from build123d import *

# Parameters (mm, degrees)
PAD_DEPTH       = 5.5
SKETCH001_R     = 1.6
POCKET_DEPTH    = 10
CHAMFER_SIZE    = 0.8
FILLET_R        = 2.49
SKETCH002_R     = 20.5
POCKET001_DEPTH = 2.5


with BuildPart() as part:
    # Sketch → Pad (new body)
    with BuildSketch(Plane.XZ):
        Polygon((0, 0), (0, -5), (5.25, -5), (5.25, -1.5), (17.75, -1.5), (17.75, -5), (23, -5), (23, 0), align=None)
    extrude(amount=PAD_DEPTH)

    # Sketch001 → Pocket (cut)
    with BuildSketch(Plane.XY):
        with Locations((2.75, -2.75)):
            Circle(SKETCH001_R)
        with Locations((20.25, -2.75)):
            Circle(SKETCH001_R)
    extrude(amount=-POCKET_DEPTH, mode=Mode.SUBTRACT)

    # Chamfer
    chamfer_edges = [part.edges().sort_by_distance(p)[0] for p in [
        (1.15, -2.75, 0),
        (18.65, -2.75, 0),
    ]]
    chamfer(chamfer_edges, length=CHAMFER_SIZE)

    # Fillet
    fillet_edges = [part.edges().sort_by_distance(p)[0] for p in [
        (0, -5.5, -2.5),
        (0, 0, -2.5),
        (23, 0, -2.5),
        (23, -5.5, -2.5),
        (5.25, -5.5, -3.25),
        (5.25, 0, -3.25),
        (17.75, -5.5, -3.25),
        (17.75, 0, -3.25),
    ]]
    fillet(fillet_edges, radius=FILLET_R)

    # Sketch002 → Pocket001 (cut)
    with BuildSketch(Plane.XY):
        with Locations((11.259596, 20)):
            Circle(SKETCH002_R)
    extrude(amount=-POCKET001_DEPTH, mode=Mode.SUBTRACT)


solid = part.part
CAD build for the part. Positions are in the model's coordinates, mm. A direction names the side the tool comes from. Round coordinates to 2 decimals unless told otherwise and drop trailing zeros. Write each loop counter-clockwise with the first axis right and the second up, starting at its lowest first coordinate (ties: lowest second). Pieces come first, ordered by that corner, then holes. Notation, with made-up numbers: M 76.25,-34 L 90.25,-34 A17 ccw 90.25,-20 Z; hole C -1,24 d2. An arc over 180 degrees is marked long. Use a Markdown table: item, result. Add a question column.
1. Slice it at C-C on z = -0.5. Give the cut face in (x, y), then the cut area to 3 significant figures.
2. 3-axis set-ups, long thin cutter, end or side, ignore diameter. For faces 4 (the face through (4.5, -0.71, -3.23)), 5 (the face through (1, -1, -5)), 6 (the face through (18.5, -4.79, -3.27)): which of +Z, -Z, +X, -X, +Y, -Y reach the whole face in a straight line?
3. Slice it at B-B on z = -4.55. Give the cut face in (x, y).
4. Flat gauge pins, fed straight in: P1, Ø3, axis at x = 2.75, y = -2.75, coming from the +Z side; P2, Ø3, axis at x = 13.5, y = -2, coming from the -Z side. Where does each tip first touch, or does it go through?
5. Drill centre lines: probe 1 along Y at (x, z) = (2.75, -2.1); probe 2 along X at (y, z) = (-4.1, -2.25); probe 3 along Z at (x, y) = (17, -1.5). Where is each one in solid material? Low to high.
6. Pull direction Y, two halves, no side cores. Call faces 1 (the face through (22.29, -0.75, -2.46)), 2 (the face through (22, -4, -5)), 3 (the face through (19.07, -1.67, -2.87)): released by +Y, released by -Y, zero draft, split by the parting line, or undercut.
7. Slice it at A-A on y = -2.75. Give the cut face in (x, z).
8. Slice it at D-D on x = 15. Give the cut face in (y, z), then the cut area to 3 significant figures.
Reply:
| question | item | result |
|---|---|---|
| 1 | outline | M 0,-3.01 A2.49 ccw 2.49,-5.5 L 20.51,-5.5 A2.49 ccw 23,-3.01 L 23,-2.49 A2.49 ccw 20.51,0 L 15.76,0 A20.5 cw 6.76,0 L 2.49,0 A2.49 ccw 0,-2.49 Z; hole C 2.75,-2.75 d3.8; hole C 20.25,-2.75 d3.8 |
| 1 | area | 95.5 mm^2 |
| 2 | face 4 | -Z, +Y |
| 2 | face 5 | -Z, +X, -X, +Y, -Y |
| 2 | face 6 | -Z, -Y |
| 3 | outline | M 0,-3.01 A2.49 ccw 2.49,-5.5 L 2.76,-5.5 A2.49 ccw 5.25,-3.01 L 5.25,-2.49 A2.49 ccw 2.76,0 L 2.49,0 A2.49 ccw 0,-2.49 Z; M 17.75,-3.01 A2.49 ccw 20.24,-5.5 L 20.51,-5.5 A2.49 ccw 23,-3.01 L 23,-2.49 A2.49 ccw 20.51,0 L 20.24,0 A2.49 ccw 17.75,-2.49 Z; hole C 2.75,-2.75 d3.2; hole C 20.25,-2.75 d3.2 |
| 4 | P1 | passes through |
| 4 | P2 | stops at z = -1.5 |
| 5 | probe 1 | y = -5.5 to -4.35, -1.15 to 0 |
| 5 | probe 2 | x = 0.25 to 1.89, 3.61 to 5, 18 to 19.39, 21.11 to 22.75 |
| 5 | probe 3 | z = -1.5 to 0 |
| 6 | face 1 | released by +Y |
| 6 | face 2 | zero draft |
| 6 | face 3 | undercut |
| 7 | outline | M 0,-5 L 1.15,-5 L 1.15,-0.8 L 0.35,0 L 0,0 Z; M 4.35,-5 L 5.25,-5 L 5.25,-1.5 L 17.75,-1.5 L 17.75,-5 L 18.65,-5 L 18.65,-0.8 L 17.85,0 L 5.15,0 L 4.35,-0.8 Z; M 21.85,-5 L 23,-5 L 23,0 L 22.65,0 L 21.85,-0.8 Z |
| 8 | outline | M -5.5,-1.5 L -0.16,-1.5 L -0.16,0 L -5.5,0 Z |
| 8 | area | 8.02 mm^2 |
